Autodesk Inventor part; units mm, degrees
ref_plane "YZ Plane" through (0, 0, 0) normal (1, 0, 0) x (0, 1, 0)
ref_plane "XZ Plane" through (0, 0, 0) normal (0, 1, 0) x (-1, 0, 0)
ref_plane "XY Plane" through (0, 0, 0) normal (0, 0, 1) x (1, 0, 0)
sketch "Bulb Copy" plane through (0, 0, 0) normal (0, 0, 1) x (1, 0, 0)
  line L0 (-16.5, 55) -> (16.5, 55) construction
  line L1 (16.5, 55) -> (16.5, 0)
  line L2 (16.5, 0) -> (-16.5, 0)
  line L3 (-16.5, 0) -> (-16.5, 55)
  line L4 (-10.5, 63) -> (10.5, 63)
  line L5 (10.5, 63) -> (10.5, 55) construction
  line L6 (10.5, 55) -> (-10.5, 55) construction
  line L7 (-10.5, 55) -> (-10.5, 63) construction
  line L8 (-16.5, 55) -> (-10.5, 63)
  line L9 (10.5, 63) -> (16.5, 55)
  line L10 (0, 63) -> (0, 0)
  point P0 (0, 55)
  dimension "d0" = 33
  dimension "d1" = 55
  dimension "d2" = 21
  dimension "d3" = 63
sketch "Top Sketch" plane through (0, 0, 0) normal (0, 0, 1) x (1, 0, 0)
  line L0 (-17.5, 56) -> (17.5, 56) construction
  line L1 (17.5, 56) -> (17.5, -15) construction
  line L2 (17.5, -15) -> (-17.5, -15) construction
  line L3 (-17.5, -15) -> (-17.5, 56) construction
  line L4 (16.5, 55) -> (16.5, 0)
  line L5 (-16.5, 0) -> (-16.5, 55)
  line L6 (-19.5, 58) -> (19.5, 58) construction
  line L7 (19.5, 58) -> (19.5, -15) construction
  line L8 (19.5, -15) -> (-19.5, -15) construction
  line L9 (-19.5, -15) -> (-19.5, 58) construction
  line L10 (-22.5, 61) -> (22.5, 61) construction
  line L11 (22.5, 61) -> (22.5, -15) construction
  line L12 (22.5, -15) -> (-22.5, -15) construction
  line L13 (-22.5, -15) -> (-22.5, 61) construction
  line L14 (-10.5, 63) -> (10.5, 63)
  line L15 (-16.5, 55) -> (16.5, 55) construction
  line L16 (-22.5, 0) -> (-19.1379, 65) construction
  line L17 (22.5, 0) -> (19.1379, 65) construction
  line L18 (-19.1379, 65) -> (19.1379, 65) construction
  line L19 (-19.1379, 65) -> (0, 97.878) construction
  line L20 (0, 97.878) -> (19.1379, 65) construction
  line L21 (-16.5, 55) -> (-10.5, 63)
  line L22 (-22.4694, 0.5911) -> (-19.3883, 60.1601)
  line L23 (-16.6999, 69.1884) -> (-8.6425, 83.0307)
  line L24 (8.6425, 83.0307) -> (16.6999, 69.1884)
  line L25 (19.3883, 60.1601) -> (22.4694, 0.5911)
  arc A0 (-16.6999, 69.1884) -> (-19.3883, 60.1601) centre (0.585, 59.127) ccw
  arc A1 (19.3883, 60.1601) -> (16.6999, 69.1884) centre (-0.585, 59.127) ccw
  arc A2 (8.6425, 83.0307) -> (-8.6425, 83.0307) centre (0, 78) ccw
  line L26 (-22.4606, -0.5906) -> (-21.7499, -11.251)
  line L27 (22.4606, -0.5906) -> (21.5, -15)
  arc A3 (-22.4694, 0.5911) -> (-22.4606, -0.5906) centre (-12.4828, 0.0746) ccw
  arc A4 (22.4606, -0.5906) -> (22.4694, 0.5911) centre (12.4828, 0.0746) ccw
  line L28 (-17.5, 56) -> (-11.0463, 64.605)
  line L29 (-10.75, 65) -> (10.75, 65) construction
  line L30 (11.0463, 64.605) -> (17.5, 56)
  line L31 (10.5, 63) -> (16.5, 55)
  line L32 (0, -15) -> (0, 88) construction
  line L33 (17.5, -8) -> (-17.5, -8)
  line L34 (-17.5, 56) -> (-17.5, -8)
  line L35 (17.5, 56) -> (17.5, -8)
  line L36 (0, 88) -> (0, -15)
  line L37 (10.75, 65) -> (0, 76.7219) construction
  line L38 (0, 76.7219) -> (-10.75, 65) construction
  line L39 (10.4163, 65.3639) -> (7.37, 68.6856)
  line L40 (-7.37, 68.6856) -> (-10.4163, 65.3639)
  arc A5 (11.0463, 64.605) -> (10.4163, 65.3639) centre (3.0463, 58.605) ccw
  arc A6 (-10.4163, 65.3639) -> (-11.0463, 64.605) centre (-3.0463, 58.605) ccw
  arc A7 (7.37, 68.6856) -> (-7.37, 68.6856) centre (0, 61.9267) ccw
  line L41 (-17, 0) -> (-17, -31.7952) construction
  line L42 (-17, -31.7952) -> (17, -31.7952) construction
  line L43 (17, -31.7952) -> (17, 0) construction
  line L44 (14.5, 12.1752) -> (-14.5, 12.1752) construction
  line L45 (6.5, 0) -> (-6.5, 0) construction
  line L46 (-6.5, 0) -> (-6.5, -30) construction
  line L47 (-6.5, -30) -> (6.5, -30) construction
  line L48 (6.5, -30) -> (6.5, 0) construction
  line L49 (-6.5, -30) -> (-18.8432, -17.6568) construction
  arc A8 (-21.7499, -11.251) -> (-20.7451, -15) centre (-11.7721, -10.5858) ccw
  line L50 (0, -15) -> (-20.7451, -15)
  point P0 (0, 0)
  point P1 (-21.5, -15)
  point P2 (0, -8)
  point P3 (0, 65)
  point P4 (0, 71.9267)
  point P5 (0, 0)
  point P6 (0, -10)
  point P7 (0, 0)
  point P8 (0, 12.1752)
  dimension "d4" = 1
  dimension "d5" = 2
  dimension "d6" = 3
  dimension "d7" = 15
  dimension "d9" = 1
  dimension "d10" = 2
  dimension "d11" = 3
  dimension "d13" = 2
  dimension "d14" = 20
  dimension "d15" = 20
  dimension "d16" = 10
  dimension "d17" = 1
  dimension "d18" = 1
  dimension "d19" = 10
  dimension "d20" = 10
  dimension "d22" = 8
  dimension "d39" = 33
  dimension "d42" = 10
  dimension "d43" = 10
  dimension "d44" = 10
  dimension "d45" = 34
  dimension "d46" = 29
  dimension "d56" = 88
  dimension "d64" = 13
  dimension "d65" = 30
  dimension "d66" = 10
revolve "Top" add sketch "Top Sketch" angle 360 about axis through (0, 88, 0) along (0, -1, 0) contours L22 A0 L23 A2 L36 A7 L40 A6 L28 L34 L33 L50 A8 L26 A3
sketch "Sketch6" plane through (0, -15, 0) normal (0, -1, 0) x (1, 0, 0)
  circle A0 centre (0, 0) radius 3.2051 construction
hole "Hole3" at (0, -15, 0) direction (0, 1, 0) diameter 36.3762 depth 8 tip angle 118
chamfer "Chamfer1" distance 0.5 angle 45 2 edges at (-12.3744, -6.5865, -12.3744) (12.3744, -6.5865, 12.3744)
properties part number "Upper" material "Polycarbonate, Smoke"
Geometry: final body of the model. Coordinates: model frame, mm. A direction names the side the tool comes from. Round coordinates to 2 decimals unless told otherwise and drop trailing zeros. Order: outer loops, then holes, each group sorted by start corner. A loop starts at its lowest first (then second) coordinate and runs counter-clockwise, first axis right, second up. Notation, with made-up numbers: M -14,-10.75 L 9,-10.75 A22 cw 9,15.25 Z; hole C 84.25,74.25 d8. An arc over 180 degrees is marked long. Use one line per item in the form item = value. Start each with the question number.
Q1. Access query for faces 4 (the face through (1.983, 82.165, 8.929)), 5 (the face through (11.07, -10.94, 14.43)). Directions: +Z, -Z, +X, -X, +Y, -Y. A direction counts if a zero-diameter tool reaches every point of the face in a straight line with its end or side. Return the directions, or none.
Q2. Material intervals for line 1 (X direction, y = -11, z = 0); line 2 (X direction, y = 50, z = 8.5); line 3 (Z direction, x = 0, y = -9), sorted ascending. Write a range as [from, to].
Q3. Pin query (flat end, axial travel): pin 1 Ø1 at (x, y) = (13.5, 15) entering from +Z; pin 2 Ø1.5 at (x, y) = (11, 24) entering from -Z; pin 3 Ø2 at (x, y) = (-6.5, 72.5) entering from +Z. Return the tip coordinate at first contact, or that it passes through.
Q4. Mould query, pull axis X, two halves, no side actions, for faces 1 (the face through (13.887, 24.522, 10.648)), 2 (the face through (-19.353, 29.959, 8.024)), 3 (the face through (0.1, -15, 18.34)). Classes: +X half, -X half, draft (parallel to the pull), parting line (faces both ways), or undercut.
Q5. Cut plane A-A (y = 40.5). Return loops of the section in (x, z), and give its area (3 significant figures).
Geometry results:
q1.face_4 = +Y
q1.face_5 = -Y
q2.line_1 = [-21.77, -18.19], [18.19, 21.77]
q2.line_2 = [-18.01, -15.3], [15.3, 18.01]
q2.line_3 = [-21.9, -18.19], [18.19, 21.9]
q3.pin_1 = 17.41
q3.pin_2 = -18.63
q3.pin_3 = 14.05
q4.face_1 = undercut
q4.face_2 = parting line
q4.face_3 = draft
q5.outline = C 0,0 d40.81; hole C 0,0 d35
q5.area = 346 mm^2
